Autodesk Inventor part; units mm, degrees
ref_plane "YZ Plane" through (0, 0, 0) normal (1, 0, 0) x (0, 1, 0)
ref_plane "XZ Plane" through (0, 0, 0) normal (0, 1, 0) x (-1, 0, 0)
ref_plane "XY Plane" through (0, 0, 0) normal (0, 0, 1) x (1, 0, 0)
sketch "Эскиз1" plane through (0, 0, 0) normal (0, 0, 1) x (1, 0, 0)
  line L0 (49.9998, 0) -> (189, 0)
  line L1 (189, 0) -> (189, -28)
  line L2 (189, -28) -> (178, -28)
  line L3 (178, -28) -> (178, -108)
  line L4 (178, -108) -> (189, -108)
  line L5 (150.5518, -43) -> (70.9998, -43)
  line L6 (54.9998, -59) -> (54.9998, -152)
  line L7 (24.9998, -84) -> (22.4998, -84)
  line L8 (22.4998, -84) -> (22.4998, -20)
  line L9 (22.4998, -20) -> (49.9998, -20)
  line L10 (49.9998, -20) -> (49.9998, 0)
  arc A0 (70.9998, -43) -> (54.9998, -59) centre (70.9998, -59) ccw
  line L11 (0, 0) -> (0, 25.6698)
  line L12 (189, -108) -> (189, -120)
  line L13 (189, -144) -> (169, -144)
  line L14 (169, -144) -> (169, -152)
  line L15 (189, -144) -> (189, -132)
  line L16 (189, -132) -> (178, -132)
  line L17 (178, -132) -> (178, -120)
  line L18 (178, -120) -> (189, -120)
  line L19 (189, -108) -> (189, -120)
  line L20 (160, -152) -> (160, -106)
  line L21 (34.9998, -144) -> (34.9998, -94)
  line L22 (169, -152) -> (160, -152)
  line L23 (54.9998, -152) -> (39.9998, -152)
  line L24 (39.9998, -152) -> (39.9998, -144)
  line L25 (39.9998, -144) -> (34.9998, -144)
  arc A1 (34.9998, -94) -> (24.9998, -84) centre (24.9998, -94) ccw
  line L26 (160, -106) -> (166.391, -61.2627)
  arc A2 (166.391, -61.2627) -> (150.5518, -43) centre (150.5518, -59) ccw
  point P0 (54.9998, -43)
  point P1 (34.9998, -98)
  dimension "d0" = 189
  dimension "d1" = 28
  dimension "d2" = 11
  dimension "d3" = 80
  dimension "d17" = 64
  dimension "d18" = 27.5
  dimension "d24" = 16
  dimension "d29" = 20
  dimension "d30" = 8
  dimension "d31" = 12
  dimension "d32" = 11
  dimension "d33" = 12
  dimension "d34" = 12
  dimension "d35" = 46
  dimension "d36" = 93
  dimension "d37" = 46
  dimension "d38" = 15
  dimension "d39" = 20
  dimension "d40" = 5
  dimension "d41" = 8
  dimension "d42" = 10
  dimension "d43" = 9
  dimension "d44" = 169
  dimension "d45" = 16
revolve "Вращение1" add sketch "Эскиз1" angle 360 about axis through (0, 0, 0) along (0, 1, 0)
properties part number "Верхняя часть поршня" material "Чугун, серый"
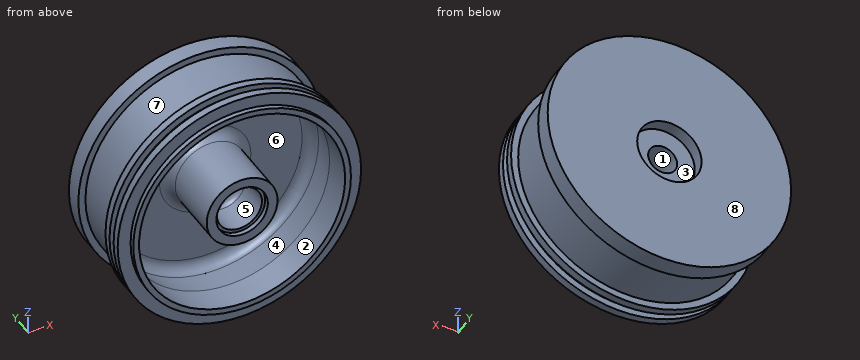
Geometry check sheet. Reference: the model listing, model coordinates, mm. Face numbers are marked on the shaded views. A direction names the side the tool comes from. Round coordinates to 2 decimals unless told otherwise and drop trailing zeros. Loops run counter-clockwise (first coordinate to the right, second up) from the corner with the lowest first, then second, coordinate; pieces in that order, holes last. Notation, with made-up numbers: (17.25, 61.5) -> (30.25, 61.5) arc R18 ccw to (30.25, 86.5) -> close; hole circle Ø6 at (6, 24.25). An arc over 180 degrees is marked (long way). Use a Markdown table: item, result.
(1) Scan lines: probe 1 along Y at (x, z) = (-152, 108.5); probe 2 along X at (y, z) = (-150, 0); probe 3 along X at (y, z) = (-12, 0). Record each from-to range of solid material in increasing order.
Calculated:
| item | result |
|---|---|
| probe 1 | -144 to -132, -120 to -108, -28 to 0 |
| probe 2 | -169 to -160, -55 to -40, 40 to 55, 160 to 169 |
| probe 3 | -189 to -50, 50 to 189 |
(2) Mould release check, pull along Y, two halves, no side actions. Record for the marked faces 5, 6, 7 and 8: released by +Y, released by -Y, zero draft, split by the parting line, or undercut.
Calculated:
| item | result |
|---|---|
| face 5 | zero draft |
| face 6 | released by -Y |
| face 7 | undercut |
| face 8 | released by +Y |
(3) Sectioned sample at B-B (y = -68). Enter the section's corners in (x, z), then the cut area to 3 significant figures.
Calculated:
| item | result |
|---|---|
| outline | circle Ø356 at (0, 0); circle Ø110 at (0, 0); hole circle Ø330.86 at (0, 0); hole circle Ø45 at (0, 0) |
| area | 21,500 mm² |
(4) Sectioned sample at A-A (y = -12.5). Enter the section's corners in (x, z).
Calculated:
| item | result |
|---|---|
| outline | circle Ø378 at (0, 0); hole circle Ø100 at (0, 0) |
(5) Set-up check for the marked faces 1, 2, 3 and 4: record each of +Z, -Z, +X, -X, +Y, -Y from which the full face is reachable in a straight line by a thin tool's end or side.
Calculated:
| item | result |
|---|---|
| face 1 | +Y, -Y |
| face 2 | -Y |
| face 3 | +Y |
| face 4 | none |
(6) Go/stop test with flat-tipped pins: P1, Ø1, axis at x = -103.5, z = -62, coming from the +Y side; P2, Ø5, axis at y = -76, z = 130, coming from the -X side; P3, Ø3, axis at y = -74, z = 67.5, coming from the -X side; P4, Ø1, axis at y = -27, z = 39, coming from the +X side. Record where each tip stops, or that it passes through.
Calculated:
| item | result |
|---|---|
| P1 | y = 0 |
| P2 | x = -124.21 |
| P3 | x = -165.31 |
| P4 | x = 185.04 |
